For this review, take the finished solid that the model builds, in its own axes (mm). Face numbers are marked on the shaded views. A direction names the side the tool comes from. Coordinates: 2 decimals unless noted, no trailing zeros. Order: outer loops, then holes, each group sorted by start corner. A loop starts at its lowest first (then second) coordinate and runs counter-clockwise, first axis right, second up. Notation, with made-up numbers: (78, 64.25) -> (126, 64.25) arc R11 ccw to (126, 80.25) -> close; hole circle Ø5 at (7.25, -24). An arc over 180 degrees is marked (long way). Return JSON: item names as keys, results as strings. Group by question number.
Item 1: Insertion check: pin 1 (7.5 mm diameter, centred on y = -5, z = 34.5, fed in from -X); pin 2 (0.8 mm diameter, centred on x = -32, y = -4, fed in from +Z); pin 3 (4.5 mm diameter, centred on y = -5, z = -13.5, fed in from +X). Each pin has a flat end and moves straight along its axis. Give the tip position at first contact, or say it passes through.
Item 2: Take a section at B-B (z = 63). Write out the cut boundary in (x, y), then the cut area to 3 significant figures.
Item 3: Machinability: for the marked faces 3 and 4, which of the approach directions +Z, -Z, +X, -X, +Y, -Y give a long, thin tool a straight path to every point of the face, cutting with its end or side? Answer none if there is none.
Item 4: For line 1 along X through (y, z) = (-5.75, -21); line 2 along X through (y, z) = (-1, 23); line 3 along Y through (x, z) = (34.25, 22), list the stretches that pass through material, from the lowest coordinate up.
Item 5: Draft analysis for pull direction Z (two halves, no side actions). For the marked faces 1 and 2, state which applies: +Z half, -Z half, draft (parallel to the pull), parting line (faces both ways), or undercut.
Item 6: Take a section at A-A (z = -55). Write out the cut boundary in (x, y).
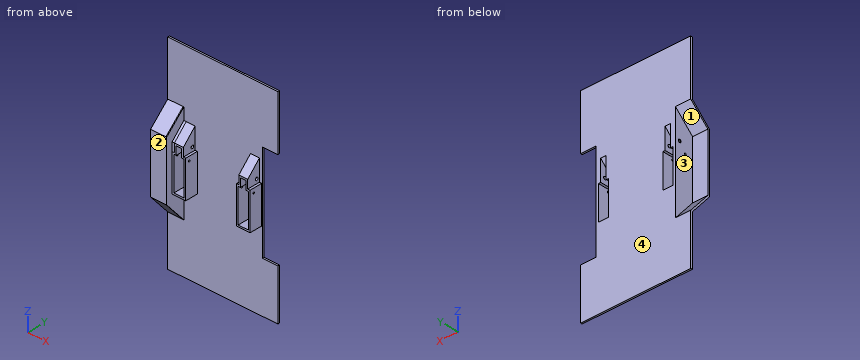
```python
from build123d import *
from build123d.topology import SkipClean

# Parameters (mm, degrees)
SKETCH1_W                = 100
SKETCH1_H                = 100
BOSS_EXTRUDE1_DEPTH      = 2
CUT_EXTRUDE1_REACH       = 72.739
SKETCH2_W                = 12
SKETCH2_H                = 50
SKETCH3_W                = 2.75
SKETCH3_H                = 10
BOSS_EXTRUDE2_DEPTH      = 2
BOSS_EXTRUDE3_DEPTH      = 15
SKETCH5_R                = 1.75
SKETCH5_R_2              = 1
CUT_EXTRUDE2_DEPTH       = 103.318131336
CHAMFER1_SIZE            = 15
CHAMFER1_OF_MIRROR1_SIZE = 15
SKETCH6_W                = 130
SKETCH6_H                = 240
SKETCH6_W_2              = 100
SKETCH6_H_2              = 100
BOSS_EXTRUDE4_DEPTH      = 2
CUT_EXTRUDE3_REACH       = 139.295
SKETCH7_W                = 18
SKETCH7_H                = 115
BOSS_EXTRUDE5_DEPTH      = 18
SKETCH9_R                = 1.75
SKETCH9_R_2              = 1
BOSS_EXTRUDE10_DEPTH     = 1
BOSS_EXTRUDE11_START     = 2.75
SKETCH10_R               = 1.75
BOSS_EXTRUDE11_DEPTH     = 2.75


with BuildPart() as part:
    # Sketch1 → Boss-Extrude1 (new body)
    with BuildSketch(Plane(origin=(0, 0, 0), x_dir=(1, 0, 0), z_dir=(0, 1, 0))):
        Rectangle(SKETCH1_W, SKETCH1_H)
    extrude(amount=BOSS_EXTRUDE1_DEPTH)

    # Sketch2 → Cut-Extrude1 (cut, up to next)
    with BuildSketch(Plane(origin=(0, 2, 0), x_dir=(1, 0, 0), z_dir=(0, 1, 0)), mode=Mode.PRIVATE) as cut_extrude1_sk1:
        with Locations((38, 0)):
            Rectangle(SKETCH2_W, SKETCH2_H)
    cut_extrude1_tool1 = extrude(cut_extrude1_sk1.sketch, amount=-CUT_EXTRUDE1_REACH, mode=Mode.PRIVATE) & part.part
    cut_extrude1 = cut_extrude1_tool1.solids().sort_by_distance((38, 2, 0))[0]
    add(cut_extrude1, mode=Mode.SUBTRACT)

    # Sketch3 → Boss-Extrude2 (add)
    with BuildSketch(Plane.XZ):
        with Locations((33.375, 20)):
            Rectangle(SKETCH3_W, SKETCH3_H)
        with Locations((42.625, 20)):
            Rectangle(SKETCH3_W, SKETCH3_H)
    boss_extrude2 = extrude(amount=-BOSS_EXTRUDE2_DEPTH)

    # Sketch4 → Boss-Extrude3 (add)
    with BuildSketch(Plane.XZ):
        Polygon((46, 17), (43.25, 17), (43.25, 27), (32.75, 27), (32.75, 17), (30, 17), (30, -27), (46, -27), align=None)
        Polygon((44, 15), (41.25, 15), (41.25, 25), (34.75, 25), (34.75, 15), (32, 15), (32, -25), (44, -25), align=None, mode=Mode.SUBTRACT)
    boss_extrude3 = extrude(amount=BOSS_EXTRUDE3_DEPTH)

    # Sketch5 → Cut-Extrude2 (cut, symmetric)
    with BuildSketch(Plane.ZY.offset(-38)):
        with Locations(Location((22, -3.5, 0), (0, 0, 180))):
            Circle(SKETCH5_R)
        with Locations((12, -10.5)):
            Circle(SKETCH5_R_2)
    cut_extrude2 = extrude(amount=CUT_EXTRUDE2_DEPTH, both=True, mode=Mode.SUBTRACT)

    # Chamfer1
    chamfer1_edges = [part.edges().sort_by_distance(p)[0] for p in [
        (38, 2, 25),
        (38, 0, 27),
    ]]
    chamfer(chamfer1_edges, length=CHAMFER1_SIZE - 0.0001)  # a hair under: the kernel refuses the full size

    # Mirror1: Cut-Extrude1, Boss-Extrude2, Boss-Extrude3, Cut-Extrude2 across plane
    add(cut_extrude1.mirror(Plane(origin=(0, 0, 0), x_dir=(0, 0, 1), z_dir=(1, 0, 0))), mode=Mode.SUBTRACT)
    add(boss_extrude2.mirror(Plane(origin=(0, 0, 0), x_dir=(0, 0, 1), z_dir=(1, 0, 0))))
    add(boss_extrude3.mirror(Plane(origin=(0, 0, 0), x_dir=(0, 0, 1), z_dir=(1, 0, 0))))
    add(cut_extrude2.mirror(Plane(origin=(0, 0, 0), x_dir=(0, 0, 1), z_dir=(1, 0, 0))), mode=Mode.SUBTRACT)

    # Chamfer1 of Mirror1
    chamfer1_of_mirror1_edges = [part.edges().sort_by_distance(p)[0] for p in [
        (-38, 2, 25),
        (-38, 0, 27),
    ]]
    chamfer(chamfer1_of_mirror1_edges, length=CHAMFER1_OF_MIRROR1_SIZE - 0.0001)  # a hair under: the kernel refuses the full size

    # Sketch6 → Boss-Extrude4 (add)
    with BuildSketch(Plane.XZ):
        Rectangle(SKETCH6_W, SKETCH6_H)
        Rectangle(SKETCH6_W_2, SKETCH6_H_2, mode=Mode.SUBTRACT)
    extrude(amount=-BOSS_EXTRUDE4_DEPTH)

    # Sketch7 → Cut-Extrude3 (cut, up to next)
    with BuildSketch(Plane.XZ, mode=Mode.PRIVATE) as cut_extrude3_sk1:
        with Locations((-56, -2.5)):
            Rectangle(SKETCH7_W, SKETCH7_H)
    cut_extrude3_tool1 = extrude(cut_extrude3_sk1.sketch, amount=-CUT_EXTRUDE3_REACH, mode=Mode.PRIVATE) & part.part
    # Sketch7 → Cut-Extrude3 (cut, up to next)
    with BuildSketch(Plane.XZ, mode=Mode.PRIVATE) as cut_extrude3_sk2:
        with Locations((56, -2.5)):
            Rectangle(SKETCH7_W, SKETCH7_H)
    cut_extrude3_tool2 = extrude(cut_extrude3_sk2.sketch, amount=-CUT_EXTRUDE3_REACH, mode=Mode.PRIVATE) & part.part
    add(cut_extrude3_tool1.solids().sort_by_distance((-56, 0, -2.5))[0], mode=Mode.SUBTRACT)
    add(cut_extrude3_tool2.solids().sort_by_distance((56, 0, -2.5))[0], mode=Mode.SUBTRACT)

    # Sketch8 → Boss-Extrude5 (add)
    with BuildSketch(Plane.ZY.offset(65)):
        Polygon((55, 2), (34.200780206, -20), (-34.200780206, -20), (-60, 2), (-61.297715069, 0.478180168), (-34.937737308, -22), (35.062262692, -22), (56.453319038, 0.62600445), align=None)
    extrude(amount=-BOSS_EXTRUDE5_DEPTH)

    # Sketch9 → Boss-Extrude10 (add)
    with BuildSketch(Plane(origin=(-47, 0, 0), x_dir=(0, 0, -1), z_dir=(1, 0, 0))):
        Polygon((63.08234072, 2), (-57.75232065, 2), (-35.062262692, -22), (34.937737308, -22), align=None)
        with Locations((-22, -3.5)):
            Circle(SKETCH9_R, mode=Mode.SUBTRACT)
        with Locations(Location((-12, -10.5, 0), (0, 0, 180))):
            Circle(SKETCH9_R_2, mode=Mode.SUBTRACT)
    extrude(amount=BOSS_EXTRUDE10_DEPTH)

    # Sketch10 → Boss-Extrude11 (add)
    with SkipClean():  # the faces are left unmerged after this step: merging them gives an invalid solid
        with BuildSketch(Plane.ZY.offset(43.25).offset(BOSS_EXTRUDE11_START)):
            Polygon((42, 0), (17, 0), (17, -15), (27, -15), align=None)
            with Locations(Location((22, -3.5, 0), (0, 0, 180))):
                Circle(SKETCH10_R, mode=Mode.SUBTRACT)
        extrude(amount=-BOSS_EXTRUDE11_DEPTH)


solid = part.part
```
Findings below:
{
 "1": {"pin 1": "stops at x = -47", "pin 2": "stops at z = 17", "pin 3": "stops at x = 46"},
 "2": {"outline": "(-65, 0) -> (65, 0) -> (65, 2) -> (-65, 2) -> close", "area": "260 mm2"},
 "3": {"face 3": "-X, +Y", "face 4": "+Z, -Z, +X, -X, +Y"},
 "4": {"line 1": "x = -47 to -44, -32 to -30, 30 to 32, 44 to 46", "line 2": "x = -47 to -41.25, -34.75 to -32.75, 32.75 to 34.75, 41.25 to 43.25", "line 3": "y = -15 to -5.25, -1.75 to 2"},
 "5": {"face 1": "undercut", "face 2": "draft"},
 "6": {"outline": "(-65, -4.89) -> (-46, -4.89) -> (-46, 0) -> (47, 0) -> (47, 2) -> (-47, 2) -> (-47, -2.26) -> (-65, -2.26) -> close"}
}
